from build123d import *

# Parameters (mm, degrees)
ENL_V_MAT_EXTRU_1_DEPTH = 4.5


with BuildPart() as part:
    # Esquisse1 → Base-Révolution (revolve)
    with BuildSketch(Plane.XY, mode=Mode.PRIVATE) as base_r_volution_sk:
        Polygon((0, 0), (0, 7.5), (1, 8.5), (38, 8.5), (38, 7), (39.5, 7), (39.5, 8.5), (49.5, 8.5), (49.5, 10), (68, 10), (68, 8.25), (69.5, 8.25), (69.5, 10), (81.5, 10), (81.5, 12.5), (88.5, 12.5), (88.5, 10), (94.5, 10), (96.5, 8), (96.5, 0), align=None)
    revolve(base_r_volution_sk.sketch.rotate(Axis((0, 0, 0), (1, 0, 0)), 90), axis=Axis((0, 0, 0), (1, 0, 0)))

    # Esquisse2 → Enlèv. mat.-Extru.1 (cut)
    with BuildSketch(Plane(origin=(0, 10, 0), x_dir=(-1, 0, 0), z_dir=(0, 1, 0))):
        with BuildLine():
            Line((-21, 2.5), (-5, 2.5))
            ThreePointArc((-5, 2.5), (-2.5, 0), (-5, -2.5))
            Line((-5, -2.5), (-21, -2.5))
            ThreePointArc((-21, -2.5), (-23.5, 0), (-21, 2.5))
        make_face()
    extrude(amount=-ENL_V_MAT_EXTRU_1_DEPTH, mode=Mode.SUBTRACT)


solid = part.part
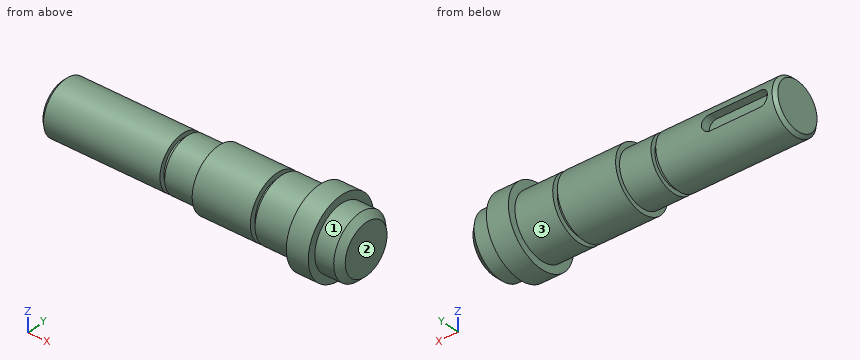
For this review, take the finished solid that the model builds, in its own axes (mm). Face numbers are marked on the shaded views. A direction names the side the tool comes from. Coordinates: 2 decimals unless noted, no trailing zeros. Loops run counter-clockwise (first coordinate to the right, second up) from the corner with the lowest first, then second, coordinate; pieces in that order, holes last. Notation, with made-up numbers: (29, 53) - (47, 53) arc R29 ccw to (47, 75) - close; hole circle Ø9 at (9.5, -39). An arc over 180 degrees is marked (long way). Use a Markdown table: item, result. Add a question column.
Item 1: Insertion check: pin 1 Ø10 at (x, z) = (36.5, -1) entering from +Y; pin 2 Ø12 at (x, z) = (80.5, -4) entering from -Y; pin 3 Ø1.5 at (x, z) = (14.5, -0.5) entering from +Y; pin 4 Ø12 at (x, y) = (12.5, -3) entering from -Z. Each pin has a flat end and moves straight along its axis. Give the tip position at first contact, or say it passes through.
Item 2: For line 1 (X direction, y = -7, z = -2.25); line 2 (X direction, y = 9, z = -4.5); line 3 (X direction, y = 4.5, z = -8.5), list the stretches that pass through material, from the lowest coordinate up.
Item 3: We need section B-B (z = 11.25). Give the boundary of the cut face in (x, y).
Item 4: Tool access review of the marked faces 1, 2 and 3: name each direction out of +Z, -Z, +X, -X, +Y, -Y from which nothing blocks a thin tool from reaching the whole face with its end or side.
Item 5: We need section A-A (x = 84). Give the boundary of the cut face in (y, z).
Results list:
| question | item | result |
|---|---|---|
| 1 | pin 1 | stops at y = 8.5 |
| 1 | pin 2 | stops at y = -12.5 |
| 1 | pin 3 | stops at y = 5.5 |
| 1 | pin 4 | stops at z = -8.5 |
| 2 | line 1 | x = 0 to 38, 39.5 to 96.5 |
| 2 | line 2 | x = 81.5 to 88.5 |
| 2 | line 3 | x = 49.5 to 68, 69.5 to 94.88 |
| 3 | outline | (81.5, -5.45) - (88.5, -5.45) - (88.5, 5.45) - (81.5, 5.45) - close |
| 4 | face 1 | +X |
| 4 | face 2 | +Z, -Z, +X, +Y, -Y |
| 4 | face 3 | -X |
| 5 | outline | circle Ø25 at (0, 0) |
